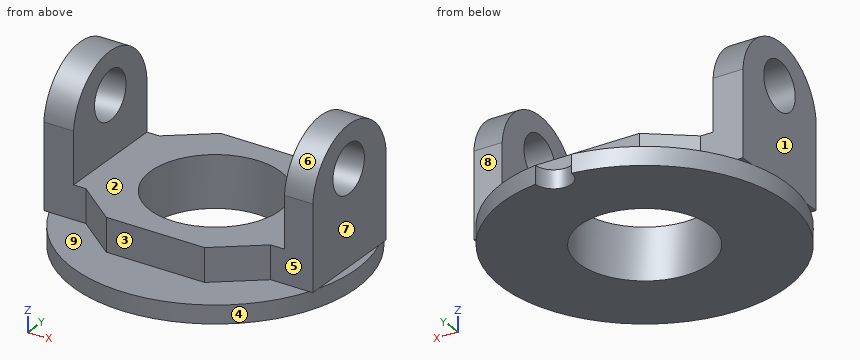
```python
from build123d import *

# Parameters (mm, degrees)
SKETCH1_R           = 10.75
BOSS_EXTRUDE1_DEPTH = 3
SKETCH2_R           = 10.75
SKETCH2_W           = 7
SKETCH2_H           = 18.67
BOSS_EXTRUDE2_DEPTH = 5.5
SKETCH3_W           = 4.95272352
SKETCH3_H           = 18.67
SKETCH3_W_2         = 4.714710678
BOSS_EXTRUDE3_DEPTH = 17
CUT_EXTRUDE1_DEPTH  = 17
SKETCH5_R           = 4
CUT_EXTRUDE2_DEPTH  = 17
CUT_EXTRUDE3_DEPTH  = 17
SKETCH7_R           = 4
CUT_EXTRUDE4_DEPTH  = 17


with BuildPart() as part:
    # Sketch1 → Boss-Extrude1 (new body)
    with BuildSketch(Plane.XY):
        with BuildLine():
            ThreePointArc((2.933453688, 23.316192859), (0.067095287, -23.499904217), (-3.066546312, 23.299062078))
            ThreePointArc((-3.066546312, 23.299062078), (-0.057980921, 20.307627469), (2.933453688, 23.316192859))
        make_face()
        Circle(SKETCH1_R, mode=Mode.SUBTRACT)
    extrude(amount=BOSS_EXTRUDE1_DEPTH)

    # Sketch2 → Boss-Extrude2 (add)
    # profile 1 of 3: a face of its own
    with BuildSketch(Plane.XY.offset(3)):
        Polygon((8.7, 14.650778086), (-8.7, 14.650778086), (-15.45272352, 9.335), (-15.45272352, -9.335), (-8.422507082, -14.869221914), (7.946481399, -14.869221914), (15.214710678, -9.147635088), (15.214710678, 9.522364912), align=None)
        Circle(SKETCH2_R, mode=Mode.SUBTRACT)
    # profile 2 of 3: a face of its own
    with BuildSketch(Plane.XY.offset(3)):
        with Locations((-18.95272352, 0)):
            Rectangle(SKETCH2_W, SKETCH2_H)
    # profile 3 of 3: a face of its own
    with BuildSketch(Plane.XY.offset(3)):
        with Locations((18.714710678, 0.187364912)):
            Rectangle(SKETCH2_W, SKETCH2_H)
    extrude(amount=BOSS_EXTRUDE2_DEPTH)

    # Sketch3 → Boss-Extrude3 (add)
    with BuildSketch(Plane.XY.offset(8.5)):
        with Locations((-19.97636176, 0)):
            Rectangle(SKETCH3_W, SKETCH3_H)
        with Locations((19.857355339, 0.187364912)):
            Rectangle(SKETCH3_W_2, SKETCH3_H)
    extrude(amount=BOSS_EXTRUDE3_DEPTH)

    # Sketch4 → Cut-Extrude1 (cut)
    with BuildSketch(Plane.ZY.offset(22.45272352)):
        with BuildLine():
            Line((17, 9.335), (17, 13.633615677))
            Line((17, 13.633615677), (31.027251007, 13.633615677))
            Line((31.027251007, 13.633615677), (31.027251007, -15.42955238))
            Line((31.027251007, -15.42955238), (17, -15.42955238))
            Line((17, -15.42955238), (17, -9.335))
            ThreePointArc((17, -9.335), (25.5, 0), (17, 9.335))
        make_face()
    extrude(amount=-CUT_EXTRUDE1_DEPTH, mode=Mode.SUBTRACT)

    # Sketch5 → Cut-Extrude2 (cut)
    with BuildSketch(Plane.ZY.offset(22.45272352)):
        with Locations((18.500000216, 0.001740409)):
            Circle(SKETCH5_R)
    extrude(amount=-CUT_EXTRUDE2_DEPTH, mode=Mode.SUBTRACT)

    # Sketch6 → Cut-Extrude3 (cut)
    with BuildSketch(Plane(origin=(22.214710678, 0, 0), x_dir=(0, 0, -1), z_dir=(1, 0, 0))):
        with BuildLine():
            Line((-17, 9.522364912), (-17, 12.0175707))
            Line((-17, 12.0175707), (-28.32322093, 12.0175707))
            Line((-28.32322093, 12.0175707), (-28.32322093, -10.554300966))
            Line((-28.32322093, -10.554300966), (-17, -10.554300966))
            Line((-17, -10.554300966), (-17, -9.147635088))
            ThreePointArc((-17, -9.147635088), (-25.5, 0.187364912), (-17, 9.522364912))
        make_face()
    extrude(amount=-CUT_EXTRUDE3_DEPTH, mode=Mode.SUBTRACT)

    # Sketch7 → Cut-Extrude4 (cut)
    with BuildSketch(Plane(origin=(22.214710678, 0, 0), x_dir=(0, 0, -1), z_dir=(1, 0, 0))):
        with Locations(Location((-18.503182636, -0.023696141, 0), (0, 0, 90))):
            Circle(SKETCH7_R)
    extrude(amount=-CUT_EXTRUDE4_DEPTH, mode=Mode.SUBTRACT)


solid = part.part
```
Could you check a few things on this model? Use its own coordinates, in mm. Face numbers are marked on the shaded views. A direction names the side the tool comes from. Give positions to 0.01 mm unless a question says otherwise; leave off trailing zeros. Write each loop counter-clockwise with the first axis right and the second up, starting at its lowest first coordinate (ties: lowest second). Pieces come first, ordered by that corner, then holes. Notation, with made-up numbers: (29.25, 35) - (45.25, 35) arc R23 ccw to (45.25, 54) - close; hole circle Ø1 at (13.5, -34.5). An arc over 180 degrees is marked (long way). One line per item, written item: value. Start each with the question number.
Item 1: Imagine slicing it at B-B, the plane x = -5. List the corners of the cut face in (y, z) for me, and give its area (3 significant figures).
Item 2: Imagine slicing it at D-D, the plane x = 20. List the corners of the cut face in (y, z) for me, and give its area (3 significant figures).
Item 3: If we mould it in two halves opening along X, with no side actions, what happens to the marked faces 1, 2, 3 and 4? For each: +X half, -X half, draft (parallel to the pull), parting line (faces both ways), or undercut.
Item 4: I'm going to push flat-ended pins straight in: pin 1 (15 mm diameter, centred on x = -6.5, y = -5.5, fed in from +Z); pin 2 (15 mm diameter, centred on y = -4.5, z = 19, fed in from -X); pin 3 (3.5 mm diameter, centred on x = 20.5, z = 7.5, fed in from -Y). Where does each tip first touch, or does it pass through?
Item 5: Which directions (+Z, -Z, +X, -X, +Y, -Y) give clear straight access to the entire face, cutting with the end or side of a thin tool? Please do the marked faces 5, 6, 7, 8 and 9.
Item 6: Imagine slicing it at C-C, the plane y = -1.5. List the corners of the cut face in (x, z) for me, and give its area (3 significant figures).
Item 7: Please list where these lines run through material, in increasing order: line 1 (Y direction, x = 0, z = 5); line 2 (X direction, y = 0, z = 12.75); line 3 (Y direction, x = 0, z = 2.25). Write a range as from..to.
Geometry says:
1. outline: (-22.96, 0) - (-9.52, 0) - (-9.52, 8.5) - (-14.87, 8.5) - (-14.87, 3) - (-22.96, 3) - close; (9.52, 0) - (22.96, 0) - (22.96, 3) - (14.65, 3) - (14.65, 8.5) - (9.52, 8.5) - close
1. area: 138 mm^2
2. outline: (-12.34, 0) - (12.34, 0) - (12.34, 3) - (9.52, 3) - (9.52, 17) arc R9.38 ccw to (-9.15, 17) - (-9.15, 3) - (-12.34, 3) - close; hole circle Ø8 at (-0.02, 18.5)
2. area: 407 mm^2
3. face 1: -X half
3. face 2: undercut
3. face 3: draft
3. face 4: parting line
4. pin 1: z = 8.5
4. pin 2: x = -22.45
4. pin 3: y = -9.15
5. face 5: +Z, +X, -Y
5. face 6: +Z, +X
5. face 7: +Z, +X, +Y, -Y
5. face 8: +Z, +X, +Y
5. face 9: +Z, -Y
6. outline: (-23.45, 0) - (-10.64, 0) - (-10.64, 8.5) - (-17.5, 8.5) - (-17.5, 14.79) - (-22.45, 14.79) - (-22.45, 3) - (-23.45, 3) - close; (-22.45, 22.21) - (-17.5, 22.21) - (-17.5, 25.38) - (-22.45, 25.38) - close; (10.64, 0) - (23.45, 0) - (23.45, 3) - (22.21, 3) - (22.21, 14.79) - (17.5, 14.79) - (17.5, 8.5) - (10.64, 8.5) - close; (17.5, 22.22) - (22.21, 22.22) - (22.21, 25.35) - (17.5, 25.35) - close
6. area: 297 mm^2
7. line 1: -14.87..-10.75, 10.75..14.65
7. line 2: -22.45..-17.5, 17.5..22.21
7. line 3: -23.5..-10.75, 10.75..20.31
